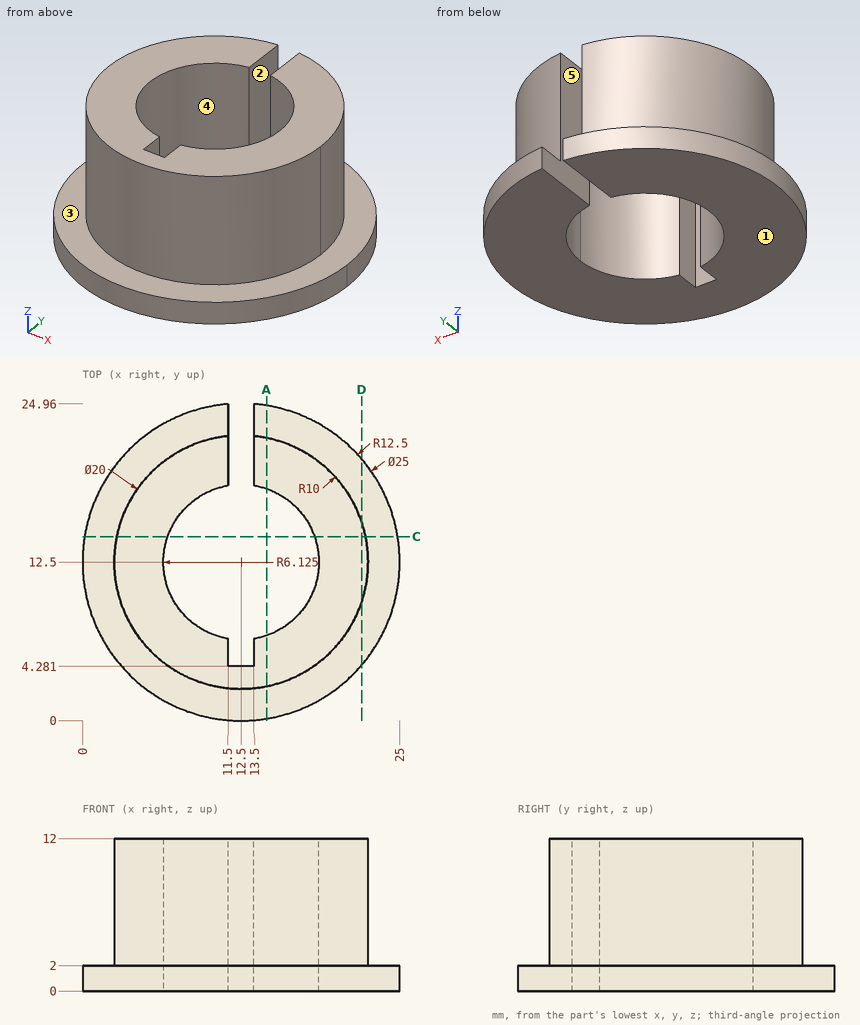
Can you work these out from the drawing? Everything is in mm from the part's minimum corner. A direction names the side the tool comes from. Coordinates: 2 decimals unless noted, no trailing zeros. Loops run counter-clockwise (first coordinate to the right, second up) from the corner with the lowest first, then second, coordinate; pieces in that order, holes last.
1) Will these pins go through, and if not, where does the flat tip stop? pin 1 Ø1.5 at (y, z) = (21.5, 6) entering from -X; pin 2 Ø2 at (x, y) = (16, 10.5) entering from -Z; pin 3 Ø2.5 at (y, z) = (5.5, 3.5) entering from +X; pin 4 Ø2 at (x, z) = (7.5, 9) entering from +Y (1 decimal).
Reported:
pin 1: stops at x = 6.85
pin 2: passes through
pin 3: stops at x = 20.68
pin 4: stops at y = 21.7
2) Imagine slicing it at A-A (x = 14.5). List the corners of the cut face in (y, z) for me, and give its area (3 significant figures).
Reported:
outline: (0.16, 0) - (6.71, 0) - (6.71, 12) - (2.7, 12) - (2.7, 2) - (0.16, 2) - close; (18.29, 0) - (24.84, 0) - (24.84, 2) - (22.3, 2) - (22.3, 12) - (18.29, 12) - close
area: 106 mm2
3) Please list where these lines run through material, in increasing order: line 1 along Z through (x, y) = (8.75, 2); line 2 along Y through (x, z) = (17, 9) (1 decimal); line 3 along X through (y, z) = (5.5, 2.75).
Reported:
line 1: z = 0 to 2
line 2: y = 3.6 to 8.3, 16.7 to 21.4
line 3: x = 5.36 to 11.5, 13.5 to 19.64
4) Imagine slicing it at D-D (x = 22). List the corners of the cut face in (y, z) for me.
Reported:
outline: (4.38, 0) - (20.62, 0) - (20.62, 2) - (15.62, 2) - (15.62, 12) - (9.38, 12) - (9.38, 2) - (4.38, 2) - close
5) Which directions (+Z, -Z, +X, -X, +Y, -Y) give clear straight access to the entire face, cutting with the end or side of a thin tool? Please do the marked faces 1, 2 and 3.
Reported:
face 1: -Z, +X, -X, +Y, -Y
face 2: +Z, -Z, +Y
face 3: +Z
6) Thinking about a two-plate mould opening in Y: for the marked faces 4 and 5, which applies, released by +Y, released by -Y, zero draft, split by the parting line, or undercut?
Reported:
face 4: undercut
face 5: zero draft
